Work out the finished part from the listing and answer in its coordinate system (mm). A direction names the side the tool comes from. Round coordinates to 2 decimals unless told otherwise and drop trailing zeros. Loops run counter-clockwise (first coordinate to the right, second up) from the corner with the lowest first, then second, coordinate; pieces in that order, holes last. Notation, with made-up numbers: M -20,42 L 21,42 A28 ccw 21,62 Z; hole C 48,-25 d3. An arc over 180 degrees is marked long. One line per item, written item: value.
```python
from build123d import *

# Parameters (mm, degrees)
F0_R     = 16
F0_R_2   = 13.35
F1_DEPTH = 15
F3_DEPTH = 25
F5_DEPTH = 25


with BuildPart() as f1:
    # F0 (on Front) → F1 (new body)
    with BuildSketch(Plane.XZ):
        Circle(F0_R)
        Circle(F0_R_2, mode=Mode.SUBTRACT)
    extrude(amount=-F1_DEPTH)

    # F2 (on Top) → F3 (cut)
    with BuildSketch(Plane.XY):
        Polygon((16, 0), (16, 15), (0, 15), (0, 12.141481), (3.25, 7.5), (0, 2.858519), (0, 0), align=None)
    extrude(amount=-F3_DEPTH, mode=Mode.SUBTRACT)

    # F4 (on Top) → F5 (cut)
    with BuildSketch(Plane.XY):
        Polygon((16, 0), (16, 15), (0, 15), (0, 12.141481), (-3.25, 7.5), (0, 2.858519), (0, 0), align=None)
    extrude(amount=F5_DEPTH, mode=Mode.SUBTRACT)


solid = f1.part
```
1) For faces 5 (the face through (0, 1, -15)), 6 (the face through (0, 1, 15)), 7 (the face through (0, 14, -15)), determine the directions among +Z, -Z, +X, -X, +Y, -Y from which every point of the face is accessible in a straight line to the end or side of a thin tool.
Check values:
face 5: +Z, -Z, +X, -Y
face 6: +Z, -Z, +X, +Y, -Y
face 7: +Z, -Z, +X, +Y
2) Find section C-C (z = 0). Give the vertices of the cut face in (x, y).
Check values:
outline: M -16,0 L -13.35,0 L -13.35,15 L -16,15 Z
3) Find the intervals of material crossed by probe 1 along X at (y, z) = (4.5, 0); probe 2 along Z at (x, y) = (-12.25, 7), in increasing order. Write a range as from..to.
Check values:
probe 1: -16..-13.35
probe 2: -10.29..-5.31, 5.31..10.29
4) Find section A-A (x = -2.5). Give the vertices of the cut face in (y, z), then the cut area to 3 significant figures.
Check values:
outline: M 0,-15.8 L 15,-15.8 L 15,-13.11 L 0,-13.11 Z; M 0,13.11 L 6.43,13.11 L 6.43,15.8 L 0,15.8 Z; M 8.57,13.11 L 15,13.11 L 15,15.8 L 8.57,15.8 Z
area: 74.9 mm2
5) The mould has two halves that part along Y. Classify faces 1 (the face through (0, 14, 15)), 2 (the face through (-1.648, 5.212, 14.453)), 3 (the face through (-13.4, 15, -2.3)), 4 (the face through (-1.602, 9.853, 14.453)): +Y half, -Y half, draft (parallel to the pull), parting line (faces both ways), or undercut.
Check values:
face 1: draft
face 2: undercut
face 3: +Y half
face 4: undercut
6) Find section D-D (x = -13). Give the vertices of the cut face in (y, z), then the cut area to 3 significant figures.
Check values:
outline: M 0,-9.33 L 15,-9.33 L 15,-3.04 L 0,-3.04 Z; M 0,3.04 L 15,3.04 L 15,9.33 L 0,9.33 Z
area: 189 mm2
7) Each of these flat-tipped pins is pushed along its axis until it touches: pin 1 (3 mm diameter, centred on y = 1, z = 14, fed in from +X); pin 2 (1.5 mm diameter, centred on x = -3.5, y = 10, fed in from +Z); pin 3 (3 mm diameter, centred on y = 2, z = -15, fed in from +X). Where does it stop, or does it pass through?
Check values:
pin 1: x = 0
pin 2: z = 15.76
pin 3: x = 0.45
8) Find section B-B (x = -5.5). Give the vertices of the cut face in (y, z).
Check values:
outline: M 0,-15.02 L 15,-15.02 L 15,-12.16 L 0,-12.16 Z; M 0,12.16 L 15,12.16 L 15,15.02 L 0,15.02 Z
